from build123d import *

# Parameters (mm, degrees)
SKETCH_1_R          = 15
EXTRUDE_1_DEPTH     = 4
EXTRUDE_2_DEPTH     = 4.5
SKETCH_3_R          = 1.95
CUT_EXTRUDE_1_DEPTH = 23.852789764
SKETCH_6_R          = 1.5
CUT_EXTRUDE_2_DEPTH = 23.852789764


with BuildPart() as part:
    # 草图1 → 凸台-拉伸1 (new body)
    with BuildSketch(Plane.XY):
        Circle(SKETCH_1_R)
    extrude(amount=EXTRUDE_1_DEPTH)

    # 草图2 → 凸台-拉伸2 (add)
    with BuildSketch(Plane.XY.offset(4)):
        Polygon((3.5, 6.062177826), (-3.5, 6.062177826), (-7, 0), (-3.5, -6.062177826), (3.5, -6.062177826), (7, 0), align=None)
    extrude(amount=EXTRUDE_2_DEPTH)

    # 草图3 → 切除-拉伸1 (cut, through all)
    with BuildSketch(Plane.XY.offset(8.5)):
        Circle(SKETCH_3_R)
    extrude(amount=-CUT_EXTRUDE_1_DEPTH, mode=Mode.SUBTRACT)

    # 草图6 → 切除-拉伸2 (cut, through all)
    with BuildSketch(Plane(origin=(0, 0, 0), x_dir=(-1, 0, 0), z_dir=(0, 0, -1))):
        with Locations((0, 12.5)):
            Circle(SKETCH_6_R)
        with Locations((12.5, 0)):
            Circle(SKETCH_6_R)
        with Locations((0, -12.5)):
            Circle(SKETCH_6_R)
        with Locations((-12.5, 0)):
            Circle(SKETCH_6_R)
    extrude(amount=-CUT_EXTRUDE_2_DEPTH, mode=Mode.SUBTRACT)


solid = part.part
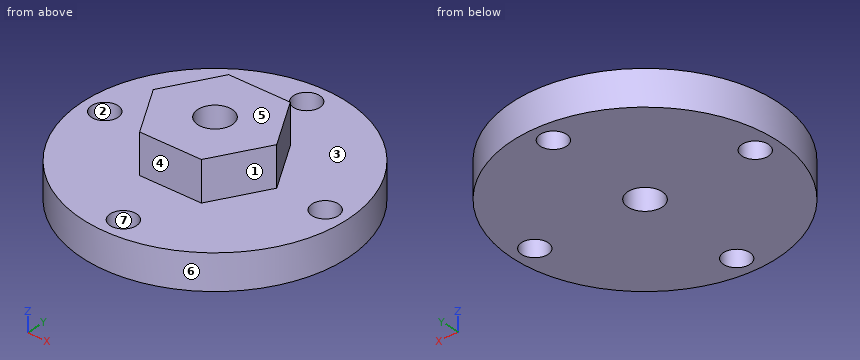
Build history of the part. All positions in model axes, mm. Face numbers are marked on the shaded views. A direction names the side the tool comes from. Coordinates: 2 decimals unless noted, no trailing zeros. Order: outer loops, then holes, each group sorted by start corner. A loop starts at its lowest first (then second) coordinate and runs counter-clockwise, first axis right, second up. Notation, with made-up numbers: (-2, -0.75) - (49, -0.75) arc R15 cw to (49, 16.25) - close; hole circle Ø11 at (-33.75, -9.5). An arc over 180 degrees is marked (long way). Write item = value, one per line. Start each with the question number.
1) 3-axis set-ups, long thin cutter, end or side, ignore diameter. For the marked faces 1, 2 and 3: which of +Z, -Z, +X, -X, +Y, -Y reach the whole face in a straight line?
2) Saw through at B-B on z = 5. Write the cut outline in (x, y), then the cut area to 3 significant figures.
3) Saw through at A-A on x = 0. Write the cut outline in (y, z), then the cut area to 3 significant figures.
4) Saw through at C-C on y = -12.5. Write the cut outline in (x, z), then the cut area to 3 significant figures.
5) Wall check: line 1 along Y through (x, z) = (-1.25, 1.5); line 2 along Z through (x, y) = (-10, -3.25); line 3 along X through (y, z) = (0.5, 3). Give the ranges that are in metal, low to high. Write a range as from..to.
6) Two-plate mould, pull along Y, no slides. Class the marked faces 4, 5, 6 and 7: pulls with the +Y half, pulls with the -Y half, needs draft (parallel to the pull), parting line crosses it, or undercut.
7) Flat gauge pins, fed straight in: pin 1 Ø3.5 at (x, y) = (0, 0) entering from +Z; pin 2 Ø3 at (x, z) = (-8.5, 3.5) entering from +Y; pin 3 Ø3.5 at (x, z) = (-1, 6.5) entering from -Y; pin 4 Ø3 at (y, z) = (1, 7) entering from +X. Where does each tip first touch, or does it go through?
From the geometry:
q1.face_1 = +Z, +X, -Y
q1.face_2 = +Z, -Z
q1.face_3 = +Z
q2.outline = (-7, 0) - (-3.5, -6.06) - (3.5, -6.06) - (7, 0) - (3.5, 6.06) - (-3.5, 6.06) - close; hole circle Ø3.9 at (0, 0)
q2.area = 115 mm^2
q3.outline = (-15, 0) - (-14, 0) - (-14, 4) - (-15, 4) - close; (-11, 0) - (-1.95, 0) - (-1.95, 8.5) - (-6.06, 8.5) - (-6.06, 4) - (-11, 4) - close; (1.95, 0) - (11, 0) - (11, 4) - (6.06, 4) - (6.06, 8.5) - (1.95, 8.5) - close; (14, 0) - (15, 0) - (15, 4) - (14, 4) - close
q3.area = 117 mm^2
q4.outline = (-8.29, 0) - (-1.5, 0) - (-1.5, 4) - (-8.29, 4) - close; (1.5, 0) - (8.29, 0) - (8.29, 4) - (1.5, 4) - close
q4.area = 54.3 mm^2
q5.line_1 = -14.95..-13.33, -11.67..-1.5, 1.5..11.67, 13.33..14.95
q5.line_2 = 0..4
q5.line_3 = -14.99..-13.91, -11.09..-1.88, 1.88..11.09, 13.91..14.99
q6.face_4 = pulls with the -Y half
q6.face_5 = needs draft
q6.face_6 = parting line crosses it
q6.face_7 = undercut
q7.pin_1 = through
q7.pin_2 = 13.27
q7.pin_3 = -6.06
q7.pin_4 = 7
